The model under review builds one solid part; all positions refer to its coordinate system, in mm. Face numbers are marked on the shaded views. A direction names the side the tool comes from. Give positions to 0.01 mm unless a question says otherwise; leave off trailing zeros. Order: outer loops, then holes, each group sorted by start corner. A loop starts at its lowest first (then second) coordinate and runs counter-clockwise, first axis right, second up.
```python
from build123d import *

# Parameters (mm, degrees)
BOSS_EXTRUDE1_DEPTH = 15
SKETCH2_W           = 30
SKETCH2_H           = 25
BOSS_EXTRUDE2_DEPTH = 10
SKETCH3_W           = 5
SKETCH3_H           = 10
CUT_EXTRUDE1_DEPTH  = 15
SKETCH6_W           = 5
SKETCH6_H           = 10
CUT_EXTRUDE4_DEPTH  = 30
SKETCH7_W           = 10
SKETCH7_H           = 10
CUT_EXTRUDE5_DEPTH  = 30


with BuildPart() as part:
    # Sketch1 → Boss-Extrude1 (new body)
    with BuildSketch(Plane.XY):
        Polygon((0, 0), (15, 0), (15, 25), (10, 25), (10, 20), (0, 10), (-10, 10), (-10, 5), (0, 5), align=None)
    extrude(amount=BOSS_EXTRUDE1_DEPTH)

    # Sketch2 → Boss-Extrude2 (add)
    with BuildSketch(Plane(origin=(0, 0, 0), x_dir=(-1, 0, 0), z_dir=(0, 0, -1))):
        with Locations((0, 12.5)):
            Rectangle(SKETCH2_W, SKETCH2_H)
    extrude(amount=BOSS_EXTRUDE2_DEPTH)

    # Sketch3 → Cut-Extrude1 (cut)
    with BuildSketch(Plane.XY):
        with Locations((-12.5, 20)):
            Rectangle(SKETCH3_W, SKETCH3_H)
    extrude(amount=-CUT_EXTRUDE1_DEPTH, mode=Mode.SUBTRACT)

    # Sketch6 → Cut-Extrude4 (cut)
    with BuildSketch(Plane.ZY.offset(10)):
        with Locations((-7.5, 20)):
            Rectangle(SKETCH6_W, SKETCH6_H)
    extrude(amount=-CUT_EXTRUDE4_DEPTH, mode=Mode.SUBTRACT)

    # Sketch7 → Cut-Extrude5 (cut)
    with BuildSketch(Plane.ZY.offset(10)):
        with Locations((5, 20)):
            Rectangle(SKETCH7_W, SKETCH7_H)
    extrude(amount=-CUT_EXTRUDE5_DEPTH, mode=Mode.SUBTRACT)


solid = part.part
```
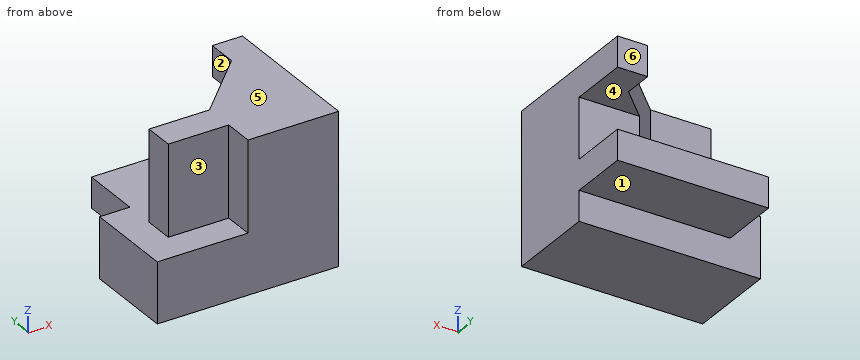
1. Take a section at C-C (x = 7.25). Write out the cut boundary in (y, z).
2. For the marked faces 1, 2 and 3, list the 3-axis set-ups (+Z, -Z, +X, -X, +Y, -Y) from which the entire face can be reached by the end or side of a thin tool; tool diameter is ignored.
3. Insertion check: pin 1 (4 mm diameter, centred on y = 8, z = 7, fed in from -X); pin 2 (8 mm diameter, centred on x = -7.5, z = 5.5, fed in from +Y); pin 3 (3 mm diameter, centred on y = 16, z = 8.5, fed in from -X). Each pin has a flat end and moves straight along its axis. Give the tip position at first contact, or say it passes through.
4. Take a section at A-A (y = 17). Write out the cut boundary in (x, z).
5. Take a section at D-D (y = 22.5). Write out the cut boundary in (x, z).
6. To check wall thickness, follow line 1 (Y direction, x = 3.5, z = -7.5); line 2 (Z direction, x = -11.5, y = 13); line 3 (Z direction, x = -3.5, y = 20). State the ranges of each line that lie inside material, in increasing order.
7. Take a section at B-B (z = 10.5). Write out the cut boundary in (x, y), and give its area (3 significant figures).
8. Draft analysis for pull direction Z (two halves, no side actions). For the marked faces 4, 5 and 6, state which applies: pulls with the +Z half, pulls with the -Z half, needs draft (parallel to the pull), parting line crosses it, or undercut.
Answer:
1. outline: (0, -10) - (15, -10) - (15, -5) - (25, -5) - (25, 0) - (15, 0) - (15, 10) - (17.25, 10) - (17.25, 15) - (0, 15) - close
2. face 1: -Z, +X, -X, +Y
2. face 2: +Z, -X, +Y
2. face 3: +Z, -X, -Y
3. pin 1: stops at x = -10
3. pin 2: stops at y = 10
3. pin 3: stops at x = 4.5
4. outline: (-10, -5) - (15, -5) - (15, 0) - (-10, 0) - close; (7, 10) - (15, 10) - (15, 15) - (7, 15) - close
5. outline: (-10, -5) - (15, -5) - (15, 0) - (-10, 0) - close; (10, 10) - (15, 10) - (15, 15) - (10, 15) - close
6. line 1: y = 0 to 15
6. line 2: z = -10 to 0
6. line 3: z = -5 to 0
7. outline: (-10, 5) - (0, 5) - (0, 0) - (15, 0) - (15, 25) - (10, 25) - (10, 20) - (0, 10) - (-10, 10) - close
7. area: 325 mm2
8. face 4: undercut
8. face 5: pulls with the +Z half
8. face 6: needs draft
